Design review of the part built by this model. Coordinates are the model's own, in mm. A direction names the side the tool comes from. Coordinates: 2 decimals unless noted, no trailing zeros. Loops run counter-clockwise (first coordinate to the right, second up) from the corner with the lowest first, then second, coordinate; pieces in that order, holes last. Notation, with made-up numbers: M 33.5,82.5 L 60.5,82.5 A15 ccw 60.5,109.5 Z; hole C -38.75,5.5 d10. An arc over 180 degrees is marked long. One line per item, written item: value.
```python
from build123d import *

# Parameters (mm, degrees)
F0_R     = 6
F0_R_2   = 10
F1_DEPTH = 6
F2_R     = 30
F2_R_2   = 10
F3_DEPTH = 13.5
F4_R     = 12
F4_R_2   = 10
F5_DEPTH = 5.5
F6_SIZE  = 1


with BuildPart() as f1:
    # F0 (on Top) → F1 (new body, symmetric)
    with BuildSketch(Plane.XY):
        with BuildLine():
            Line((-12.3333333333, 27.3475572746), (-49.7277777778, 10.4832302886))
            ThreePointArc((-49.7277777778, 10.4832302886), (-56.5, 0), (-49.7277777778, -10.4832302886))
            Line((-49.7277777778, -10.4832302886), (-12.3333333333, -27.3475572746))
            ThreePointArc((-12.3333333333, -27.3475572746), (0, -30), (12.3333333333, -27.3475572746))
            Line((12.3333333333, -27.3475572746), (49.7277777778, -10.4832302886))
            ThreePointArc((49.7277777778, -10.4832302886), (56.5, 0), (49.7277777778, 10.4832302886))
            Line((49.7277777778, 10.4832302886), (12.3333333333, 27.3475572746))
            ThreePointArc((12.3333333333, 27.3475572746), (0, 30), (-12.3333333333, 27.3475572746))
        make_face()
        with Locations((-45, 0)):
            Circle(F0_R, mode=Mode.SUBTRACT)
        Circle(F0_R_2, mode=Mode.SUBTRACT)
        with Locations((45, 0)):
            Circle(F0_R, mode=Mode.SUBTRACT)
    extrude(amount=F1_DEPTH, both=True)

    # F2 (on face) → F3 (join)
    with BuildSketch(Plane.XY.offset(6)):
        Circle(F2_R)
        Circle(F2_R_2, mode=Mode.SUBTRACT)
    extrude(amount=F3_DEPTH)

    # F4 (on face) → F5 (join)
    with BuildSketch(Plane.XY.offset(19.5)):
        Circle(F4_R)
        Circle(F4_R_2, mode=Mode.SUBTRACT)
    extrude(amount=F5_DEPTH)

    # F6
    f6_edges = [f1.edges().sort_by_distance(p)[0] for p in [
        (-30, 0, 19.5),
    ]]
    chamfer(f6_edges, length=F6_SIZE)


solid = f1.part
```
(1) We need section D-D on z = 16.5. State the section outline as (x, y) points.
Reply:
outline: C 0,0 d60; hole C 0,0 d20
(2) We need section B-B on x = 0. State the section outline as (y, z) points.
Reply:
outline: M -30,-6 L -10,-6 L -10,25 L -12,25 L -12,19.5 L -29,19.5 L -30,18.5 Z; M 10,-6 L 30,-6 L 30,18.5 L 29,19.5 L 12,19.5 L 12,25 L 10,25 Z
(3) We need section A-A on y = 0. State the section outline as (x, z) points, then the cut area to 3 significant figures.
Reply:
outline: M -56.5,-6 L -51,-6 L -51,6 L -56.5,6 Z; M -39,-6 L -10,-6 L -10,25 L -12,25 L -12,19.5 L -29,19.5 L -30,18.5 L -30,6 L -39,6 Z; M 10,-6 L 39,-6 L 39,6 L 30,6 L 30,18.5 L 29,19.5 L 12,19.5 L 12,25 L 10,25 Z; M 51,-6 L 56.5,-6 L 56.5,6 L 51,6 Z
area: 1,390 mm2
(4) To check wall thickness, follow line 1 along Y through (x, z) = (0, 7); line 2 along Z through (x, y) = (-34, -9); line 3 along Z through (x, y) = (-19, -20). State the ranges of each line that lie inside material, in increasing order. Write a range as [from, to].
Reply:
line 1: y = [-30, -10], [10, 30]
line 2: z = [-6, 6]
line 3: z = [-6, 19.5]
(5) Tool access review of faces 4 (the cylindrical face through (39, 0, 0)), 5 (the cylindrical face through (-11.99, 0.53, 22.21)): name each direction out of +Z, -Z, +X, -X, +Y, -Y from which nothing blocks a thin tool from reaching the whole face with its end or side.
Reply:
face 4: +Z, -Z
face 5: +Z
(6) Insertion check: pin 1 (5 mm diameter, centred on x = 20, y = 7.5, fed in from +Z); pin 2 (12 mm diameter, centred on y = -12.5, z = 5.5, fed in from -X); pin 3 (1 mm diameter, centred on y = 14.5, z = 9.5, fed in from +X). Each pin has a flat end and moves straight along its axis. Give the tip position at first contact, or say it passes through.
Reply:
pin 1: stops at z = 19.5
pin 2: stops at x = -54.49
pin 3: stops at x = 26.53
(7) Mouldability with a two-part tool opening along Y and no side actions: class faces 1 (the cylindrical face through (-2.17, -9.76, 9.28)), 2 (the cylindrical face through (-56.5, 0.2, 0.1)), 3 (the flat face through (30.769, -19.033, 0.084)) as released by +Y, released by -Y, zero draft, split by the parting line, or undercut.
Reply:
face 1: undercut
face 2: split by the parting line
face 3: released by -Y
(8) We need section C-C on z = 0. State the section outline as (x, y) points.
Reply:
outline: M -49.73,-10.48 L -12.33,-27.35 A30 ccw 12.33,-27.35 L 49.73,-10.48 A11.5 ccw 49.73,10.48 L 12.33,27.35 A30 ccw -12.33,27.35 L -49.73,10.48 A11.5 ccw Z; hole C -45,0 d12; hole C 0,0 d20; hole C 45,0 d12
